```python
from build123d import *

# Parameters (mm, degrees)
SKETCH_W     = 80
SKETCH_H     = 100
PAD_DEPTH    = 20
SKETCH001_W  = 76
SKETCH001_H  = 16
POCKET_DEPTH = 100.001
FILLET_R     = 1


with BuildPart() as part:
    # Sketch → Pad (new body)
    with BuildSketch(Plane.XY):
        with Locations((40, 50)):
            Rectangle(SKETCH_W, SKETCH_H)
    extrude(amount=PAD_DEPTH)

    # Sketch001 (on Face1 of Pad) → Pocket (cut, through all)
    with BuildSketch(Plane.XZ):
        with Locations((40.002224, 10)):
            Rectangle(SKETCH001_W, SKETCH001_H)
    extrude(amount=-POCKET_DEPTH, mode=Mode.SUBTRACT)

    # Fillet
    fillet_edges = [part.edges().sort_by_distance(p)[0] for p in [
        (0, 50, 0),
        (80, 50, 0),
        (0, 50, 20),
        (80, 50, 20),
    ]]
    fillet(fillet_edges, radius=FILLET_R)


solid = part.part
```
Source: CAD feature listing. Evaluate the final solid. Frame: model axes, mm. A direction names the side the tool comes from. Round coordinates to 2 decimals unless told otherwise and drop trailing zeros. Order: outer loops, then holes, each group sorted by start corner. A loop starts at its lowest first (then second) coordinate and runs counter-clockwise, first axis right, second up. Notation, with made-up numbers: (70, -27.75) -> (123, -27.75) arc R13 cw to (123, -21.75) -> close; hole circle Ø3 at (-32.75, 54). An arc over 180 degrees is marked (long way). One line per item, written item: value. Start each with the question number.
Q1. Section query A-A (x = 70). Return the cut outline in (y, z).
Q2. Access query for faces 1 (the flat face through (0, 49, 10)), 2 (the flat face through (39, 49, 2)). Directions: +Z, -Z, +X, -X, +Y, -Y. A direction counts if a zero-diameter tool reaches every point of the face in a straight line with its end or side. Return the directions, or none.
Q3. Pin query (flat end, axial travel): pin 1 (10 mm diameter, centred on x = 11, z = 9.5, fed in from -Y). Return the tip coordinate at first contact, or that it passes through.
Q4. Section query B-B (y = 28.5). Return the cut outline in (x, z), plus the area to 3 significant figures.
Q5. Section query C-C (z = 8.75). Return the cut outline in (x, y), plus the area to 3 significant figures.
Q6. Material intervals for probe 1 along Z at (x, y) = (35.5, 31.5); probe 2 along X at (y, z) = (11.5, 2.75), sorted ascending.
Findings below:
1. outline: (0, 0) -> (100, 0) -> (100, 2) -> (0, 2) -> close; (0, 18) -> (100, 18) -> (100, 20) -> (0, 20) -> close
2. face 1: +Z, -Z, -X, +Y, -Y
2. face 2: +Y, -Y
3. pin 1: through
4. outline: (0, 1) arc R1 ccw to (1, 0) -> (79, 0) arc R1 ccw to (80, 1) -> (80, 19) arc R1 ccw to (79, 20) -> (1, 20) arc R1 ccw to (0, 19) -> close; hole (2, 2) -> (78, 2) -> (78, 18) -> (2, 18) -> close
4. area: 383 mm²
5. outline: (0, 0) -> (2, 0) -> (2, 100) -> (0, 100) -> close; (78, 0) -> (80, 0) -> (80, 100) -> (78, 100) -> close
5. area: 400 mm²
6. probe 1: 0 to 2, 18 to 20
6. probe 2: 0 to 2, 78 to 80
